Could you check a few things on this drawing? It's one solid part, dimensions in mm from its lowest x, y, z. A direction names the side the tool comes from. Round coordinates to 2 decimals unless told otherwise and drop trailing zeros. Write each loop counter-clockwise with the first axis right and the second up, starting at its lowest first coordinate (ties: lowest second). Pieces come first, ordered by that corner, then holes. Notation, with made-up numbers: (66.5, 78.5) -> (80.5, 78.5) arc R12 cw to (80.5, 84.5) -> close; hole circle Ø9 at (75.5, -15.75). An arc over 180 degrees is marked (long way). Answer in a Markdown table with one row per item.
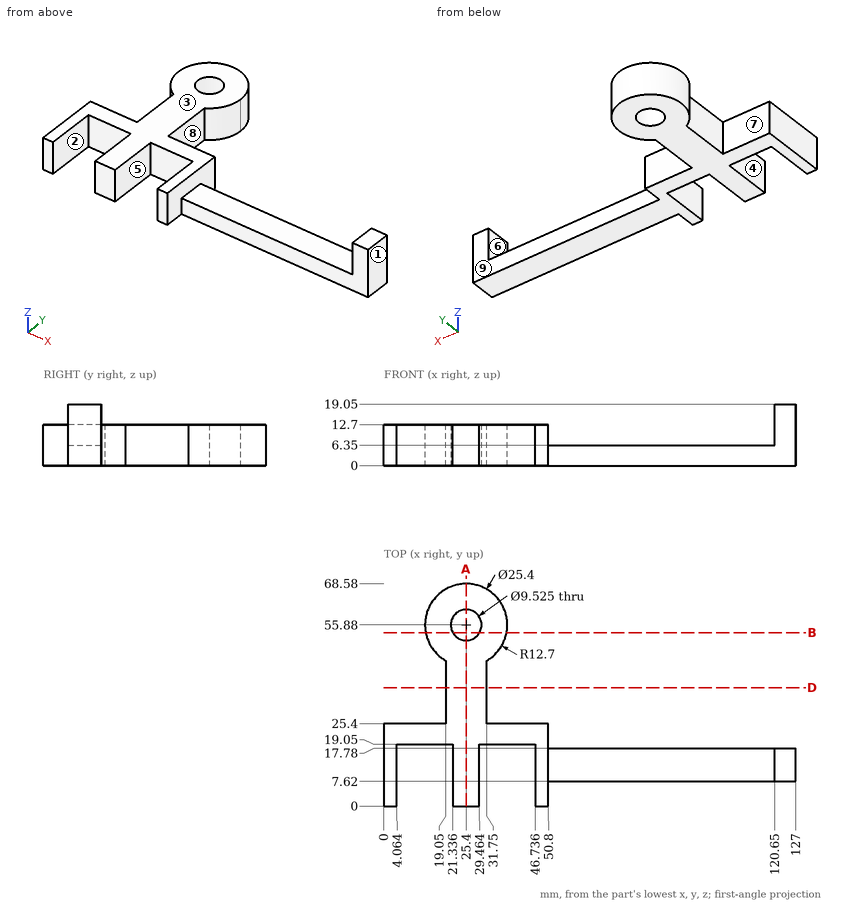
1) For pin 1 (15 mm diameter, centred on x = 30.5, y = 36, fed in from +Z); pin 2 (10 mm diameter, centred on x = 11, z = 4.5, fed in from -Y); pin 3 (8 mm diameter, centred on x = 81.5, z = 7, fed in from -Y), each with a flat end and sliding along its axis, tell me the tip position at first contact or that it passes through.
Response:
| item | result |
|---|---|
| pin 1 | stops at z = 12.7 |
| pin 2 | stops at y = 19.05 |
| pin 3 | stops at y = 7.62 |
2) We'd pull the mould along X, two halves only. Please class the marked faces 1, 2, 3 and 4: +X half, -X half, draft (parallel to the pull), parting line (faces both ways), or undercut.
Response:
| item | result |
|---|---|
| face 1 | +X half |
| face 2 | undercut |
| face 3 | draft |
| face 4 | undercut |
3) I need wall thicknesses on line 1 (Y direction, x = 25.4, z = 9); line 2 (Z direction, x = 13.5, y = 23.5); line 3 (Y direction, x = 73, z = 2.25). Which ranges of each line are inside material? Lowest first, please. Write a range as [from, to].
Response:
| item | result |
|---|---|
| line 1 | y = [0, 51.12], [60.64, 68.58] |
| line 2 | z = [0, 12.7] |
| line 3 | y = [7.62, 17.78] |
4) I want a section at B-B, the plane y = 53.5. List the corners of the cut face in (x, z) for me (3 decimals).
Response:
| item | result |
|---|---|
| outline | (12.925, 0) -> (21.275, 0) -> (21.275, 12.7) -> (12.925, 12.7) -> close; (29.525, 0) -> (37.875, 0) -> (37.875, 12.7) -> (29.525, 12.7) -> close |
5) Which directions (+Z, -Z, +X, -X, +Y, -Y) give clear straight access to the entire face, cutting with the end or side of a thin tool? Please do the marked faces 5, 6, 7, 8 and 9.
Response:
| item | result |
|---|---|
| face 5 | +Z, -Z, -Y |
| face 6 | +Z, +Y, -Y |
| face 7 | +Z, -Z, -X |
| face 8 | +Z, -Z, +X |
| face 9 | +Z, -Z, +X, +Y |
6) I want a section at D-D, the plane y = 36.5. List the corners of the cut face in (x, z) for me, and give its area (3 significant figures).
Response:
| item | result |
|---|---|
| outline | (19.05, 0) -> (31.75, 0) -> (31.75, 12.7) -> (19.05, 12.7) -> close |
| area | 161 mm^2 |
7) I want a section at A-A, the plane x = 25.4. List the corners of the cut face in (y, z) for me.
Response:
| item | result |
|---|---|
| outline | (0, 0) -> (51.12, 0) -> (51.12, 12.7) -> (0, 12.7) -> close; (60.64, 0) -> (68.58, 0) -> (68.58, 12.7) -> (60.64, 12.7) -> close |
